from build123d import *

# Parameters (mm, degrees)
SKETCH3_W            = 31.1
SKETCH3_H            = 32.1
SHELL_DEPTH          = 10
SKETCH4_W            = 27.1
SKETCH4_H            = 26.1
MAIN_CAVITY_DEPTH    = 8
SKETCH5_W            = 27.1
SKETCH5_H            = 2
SUPPORT_SHELF_DEPTH  = 6
SKETCH6_W            = 4.8
SKETCH6_H            = 7.7
SKETCH6_W_2          = 7.4
SKETCH6_W_3          = 9.5
SKETCH6_H_2          = 10
TERMINAL_INPUT_DEPTH = 2
SKETCH7_W            = 2
SKETCH7_H            = 2
MALE_TABS_DEPTH      = 2
SKETCH8_W            = 2
SKETCH8_H            = 2
CUT_EXTRUDE4_DEPTH   = 2


with BuildPart() as part:
    # Sketch3 → Shell (new body)
    with BuildSketch(Plane(origin=(0, 0, 0), x_dir=(1, 0, 0), z_dir=(0, 1, 0))):
        with Locations((15.55, -16.05)):
            Rectangle(SKETCH3_W, SKETCH3_H)
    extrude(amount=SHELL_DEPTH)

    # Sketch4 → Main Cavity (cut)
    with BuildSketch(Plane(origin=(0, 10, 0), x_dir=(1, 0, 0), z_dir=(0, 1, 0))):
        with Locations((15.55, -17.05)):
            Rectangle(SKETCH4_W, SKETCH4_H)
    extrude(amount=-MAIN_CAVITY_DEPTH, mode=Mode.SUBTRACT)

    # Sketch5 → Support Shelf (cut)
    with BuildSketch(Plane(origin=(0, 10, 0), x_dir=(1, 0, 0), z_dir=(0, 1, 0))):
        with Locations((15.55, -3)):
            Rectangle(SKETCH5_W, SKETCH5_H)
    extrude(amount=-SUPPORT_SHELF_DEPTH, mode=Mode.SUBTRACT)

    # Sketch6 → Terminal Input (cut)
    with BuildSketch(Plane.XY.offset(32.1)):
        with Locations((25.7, 6.15)):
            Rectangle(SKETCH6_W, SKETCH6_H)
        with Locations((17.9, 6.15)):
            Rectangle(SKETCH6_W_2, SKETCH6_H)
        with Locations((7.45, 5)):
            Rectangle(SKETCH6_W_3, SKETCH6_H_2)
    extrude(amount=-TERMINAL_INPUT_DEPTH, mode=Mode.SUBTRACT)

    # Sketch7 → Male Tabs (add)
    with BuildSketch(Plane(origin=(0, 10, 0), x_dir=(1, 0, 0), z_dir=(0, 1, 0))):
        with Locations((30.1, -26.112988121)):
            Rectangle(SKETCH7_W, SKETCH7_H)
        with Locations((1, -4.859742299)):
            Rectangle(SKETCH7_W, SKETCH7_H)
    extrude(amount=MALE_TABS_DEPTH)

    # Sketch8 → Cut-Extrude4 (cut)
    with BuildSketch(Plane(origin=(0, 10, 0), x_dir=(1, 0, 0), z_dir=(0, 1, 0))):
        with Locations((30.1, -4.859742299)):
            Rectangle(SKETCH8_W, SKETCH8_H)
        with Locations((1, -26.112988121)):
            Rectangle(SKETCH8_W, SKETCH8_H)
    extrude(amount=-CUT_EXTRUDE4_DEPTH, mode=Mode.SUBTRACT)


solid = part.part
The listing builds one solid part. Answer for the finished solid, in the listing's coordinates (mm). A direction names the side the tool comes from. Coordinates: 2 decimals unless noted, no trailing zeros. Order: outer loops, then holes, each group sorted by start corner. A loop starts at its lowest first (then second) coordinate and runs counter-clockwise, first axis right, second up. Notation, with made-up numbers: M 70,-21.5 L 125,-21.5 A36 ccw 125,14.5 Z; hole C 28.5,15.25 d1. An arc over 180 degrees is marked long. Use CSV: the item, a comma, the result in double quotes.
Q1. Section D-D (x = 22) is taken. Determine the outline of the cut face in (y, z).
Here are the results:
outline,"M 0,0 L 10,0 L 10,2 L 4,2 L 4,4 L 2,4 L 2,30.1 L 10,30.1 L 10,32.1 L 0,32.1 Z"
Q2. Straight lines are drawn through the part: L1, parallel to X at y = 3, z = 11; L2, parallel to Z at x = 29, y = 7.5; L3, parallel to Z at x = 20.5, y = 2.25. For each, find the intervals that lie inside material, in ascending order.
Here are the results:
L1,"0 to 2, 29.1 to 31.1"
L2,"0 to 2, 30.1 to 32.1"
L3,"0 to 4, 30.1 to 32.1"
Q3. A tool of negligible diameter and unlimited length cuts with its end or side. For faces 1 (the flat face through (26, 2.3, 31)), 2 (the flat face through (1, 9, 27.113)), 3 (the flat face through (15, 2, 17)), 4 (the flat face through (7, 1, 30.1)), 5 (the flat face through (1, 10, 30)), from which of +Z, -Z, +X, -X, +Y, -Y can it reach the whole face along a straight path? Write none if from no direction.
Here are the results:
face 1,"+Z, +Y"
face 2,"-X, +Y"
face 3,"+Y"
face 4,"+Z, +Y, -Y"
face 5,"+Z, +X, -X, +Y"
Q4. Section B-B (z = 30.5) is taken. Determine the outline of the cut face in (x, y).
Here are the results:
outline,"M 0,0 L 2.7,0 L 2.7,10 L 0,10 Z; M 12.2,0 L 31.1,0 L 31.1,10 L 28.1,10 L 28.1,2.3 L 23.3,2.3 L 23.3,10 L 21.6,10 L 21.6,2.3 L 14.2,2.3 L 14.2,10 L 12.2,10 Z"
Q5. Determine the mould class of faces 6 (the flat face through (30, 8, 5)), 7 (the flat face through (15, 7, 2)) for opening direction X: pulls with the +X half, pulls with the -X half, needs draft (parallel to the pull), parting line crosses it, or undercut.
Here are the results:
face 6,"needs draft"
face 7,"undercut"
Q6. Section A-A (y = 6.25) is taken. Determine the outline of the cut face in (x, z), then the cut area to 3 significant figures.
Here are the results:
outline,"M 0,0 L 31.1,0 L 31.1,32.1 L 28.1,32.1 L 28.1,30.1 L 29.1,30.1 L 29.1,2 L 2,2 L 2,30.1 L 2.7,30.1 L 2.7,32.1 L 0,32.1 Z; M 12.2,30.1 L 14.2,30.1 L 14.2,32.1 L 12.2,32.1 Z; M 21.6,30.1 L 23.3,30.1 L 23.3,32.1 L 21.6,32.1 Z"
area,"193 mm2"
Q7. Section C-C (y = 10.5) is taken. Determine the outline of the cut face in (x, z), then the cut area to 3 significant figures.
Here are the results:
outline,"M 0,3.86 L 2,3.86 L 2,5.86 L 0,5.86 Z; M 29.1,25.11 L 31.1,25.11 L 31.1,27.11 L 29.1,27.11 Z"
area,"8.00 mm2"
Q8. Given pin 1 Ø1.6 at (x, z) = (13, 31) entering from +Y; pin 2 Ø1.6 at (x, z) = (1.5, 26) entering from +Y; pin 3 Ø1.6 at (x, z) = (19.5, 31.5) entering from +Y, each flat-ended and moving along its own axis, determine where each tip first touches the part or whether it passes through.
Here are the results:
pin 1,"y = 10"
pin 2,"y = 8"
pin 3,"y = 2.3"
